Input: part model. Units: mm. Frame: model coordinates. A direction names the side the tool comes from. Give positions to 0.01 mm unless a question says otherwise; leave off trailing zeros. Loops run counter-clockwise (first coordinate to the right, second up) from the corner with the lowest first, then second, coordinate; pieces in that order, holes last. Notation, with made-up numbers: (5, 29.5) - (36, 29.5) arc R27 cw to (36, 68.5) - close; hole circle Ø10 at (68.5, 60.25). An arc over 180 degrees is marked (long way). Answer as a JSON object with one key per item and string values. Group by question number.
(1) Access query for faces 4 (the flat face through (18, -34.692, -36)), 5 (the flat face through (18, -5.08, -35)), 6 (the flat face through (18, -20, -7.968)). Directions: +Z, -Z, +X, -X, +Y, -Y. A direction counts if a zero-diameter tool reaches every point of the face in a straight line with its end or side. Return the directions, or none.
(2) Section query B-B (y = -32.5). Return loops of the section in (x, z).
(3) Section query A-A (z = -9). Return loops of the section in (x, y).
(4) Section query C-C (x = 21). Return loops of the section in (y, z).
(5) Mould query, pull axis Z, two halves, no side actions, for faces 1 (the flat face through (18, -20, -63.064)), 2 (the flat face through (6, -39.878, -35)), 3 (the flat face through (6, -20, 0)). Classes: +Z half, -Z half, draft (parallel to the pull), parting line (faces both ways), or undercut.
(6) Pin query (flat end, axial travel): P1, Ø3, axis at x = 16, y = -22, coming from the -Z side; P2, Ø3, axis at x = 18, z = -36.5, coming from the -Y side. Return the tip coordinate at first contact, or that it passes through.
(7) Material intervals for L1, parallel to X at y = -5, z = -18.5; L2, parallel to Z at x = 13.75, y = -27.5; L3, parallel to Y at x = 20.25, z = -56, sorted ascending.
Autodesk Inventor part; units mm, degrees
ref_plane "YZ Plane" through (0, 0, 0) normal (1, 0, 0) x (0, 1, 0)
ref_plane "XZ Plane" through (0, 0, 0) normal (0, 1, 0) x (-1, 0, 0)
ref_plane "XY Plane" through (0, 0, 0) normal (0, 0, 1) x (1, 0, 0)
sketch "Sketch1" plane through (0, 0, 0) normal (1, 0, 0) x (0, 1, 0)
  line L0 (0, 0) -> (-39.878, 0)
  line L1 (-39.878, 0) -> (-39.878, -70.104)
  line L2 (-39.878, -70.104) -> (0, -70.104)
  line L3 (0, -70.104) -> (0, 0)
  dimension "d0" = 39.878
  dimension "d1" = 70.104
extrude "Extrusion1" add sketch "Sketch1" along normal blind 12.7
sketch "Sketch2" plane through (12.7, 0, 0) normal (1, 0, 0) x (0, 0, -1)
  line L0 (7.9684, 0) -> (7.9684, -5.08) construction
  line L1 (34.6892, -39.7724) -> (34.6892, -34.6924) construction
  line L2 (34.6892, -39.7724) -> (39.7692, -39.7724) construction
  line L3 (7.9684, -5.08) -> (63.0635, -5.08)
  line L4 (63.0635, -5.08) -> (63.0635, -34.6924)
  line L5 (63.0635, -34.6924) -> (7.9684, -34.6924)
  line L6 (7.9684, -34.6924) -> (7.9684, -5.08)
  point P0 (0, 0)
  dimension "d4" = 5.08
  dimension "d5" = 5.08
  dimension "d6" = 90
extrude "Extrusion2" add sketch "Sketch2" along normal blind 10.16
properties part number "Periph_Screen"
Recorded:
{
 "1": {"face 4": "+Z, -Z, +X, -Y", "face 5": "+Z, -Z, +X, +Y", "face 6": "+Z, +X, +Y, -Y"},
 "2": {"outline": "(0, -70.1) - (12.7, -70.1) - (12.7, -63.06) - (22.86, -63.06) - (22.86, -7.97) - (12.7, -7.97) - (12.7, 0) - (0, 0) - close"},
 "3": {"outline": "(0, -39.88) - (12.7, -39.88) - (12.7, -34.69) - (22.86, -34.69) - (22.86, -5.08) - (12.7, -5.08) - (12.7, 0) - (0, 0) - close"},
 "4": {"outline": "(-34.69, -63.06) - (-5.08, -63.06) - (-5.08, -7.97) - (-34.69, -7.97) - close"},
 "5": {"face 1": "-Z half", "face 2": "draft", "face 3": "+Z half"},
 "6": {"P1": "stops at z = -63.06", "P2": "stops at y = -34.69"},
 "7": {"L1": "x = 0 to 12.7", "L2": "z = -63.06 to -7.97", "L3": "y = -34.69 to -5.08"}
}
